Here's how the part is built. I have some questions about the finished solid (model axes, mm). Give positions to 0.01 mm unless a question says otherwise; leave off trailing zeros. Order: outer loops, then holes, each group sorted by start corner. A loop starts at its lowest first (then second) coordinate and runs counter-clockwise, first axis right, second up. Notation, with made-up numbers: (12, 68.5) - (52, 68.5) arc R18 ccw to (52, 72.5) - close; hole circle Ø7 at (80.25, -22). An arc over 180 degrees is marked (long way). One line per question, with ' | ' between items.
from build123d import *

# Parameters (mm, degrees)
F0_W     = 111.695483
F0_H     = 93.271062
F1_DEPTH = 38.75114
F2_SIZE  = 12.7
F3_W     = 73.332176
F3_H     = 55.99878
F4_DEPTH = 6.398048


with BuildPart() as f1:
    # F0 (on Top) → F1 (new body)
    with BuildSketch(Plane.XY):
        with Locations((12.841567, 46.635531)):
            Rectangle(F0_W, F0_H)
    extrude(amount=-F1_DEPTH)

    # F2
    f2_edges = [f1.edges().sort_by_distance(p)[0] for p in [
        (68.689309, 46.635531, -38.75114),
    ]]
    chamfer(f2_edges, length=F2_SIZE)

    # F3 (on face) → F4 (join)
    with BuildSketch(Plane(origin=(0, 0, -38.75114), x_dir=(1, 0, 0), z_dir=(0, 0, -1))):
        with Locations((-1.400314, -35.273772)):
            Rectangle(F3_W, F3_H)
    extrude(amount=F4_DEPTH)


solid = f1.part
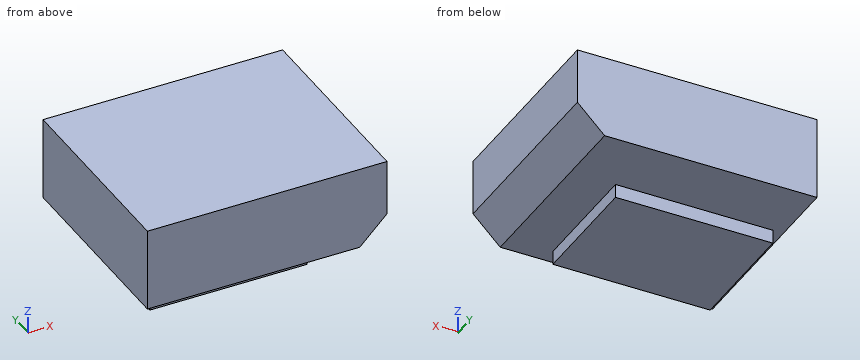
1) I'm going to push flat-ended pins straight in: P1, Ø12, axis at y = 43, z = -39.5, coming from the +X side; P2, Ø5, axis at x = -17, z = -43.5, coming from the +Y side; P3, Ø3, axis at y = 27, z = -41.5, coming from the +X side. Where does each tip first touch, or does it pass through?
Model answer:
P1: stops at x = 61.24 | P2: stops at y = 63.27 | P3: stops at x = 35.27
2) Please list where these lines run through material, in increasing order: L1, parallel to Y at x = 34, z = -41; L2, parallel to Z at x = 42.5, y = 40; L3, parallel to X at y = 47, z = -41.
Model answer:
L1: y = 7.27 to 63.27 | L2: z = -38.75 to 0 | L3: x = -38.07 to 35.27
3) I want a section at A-A (y = 10). List the corners of the cut face in (x, z) for me.
Model answer:
outline: (-43.01, -38.75) - (-38.07, -38.75) - (-38.07, -45.15) - (35.27, -45.15) - (35.27, -38.75) - (55.99, -38.75) - (68.69, -26.05) - (68.69, 0) - (-43.01, 0) - close
4) I want a section at D-D (y = 84). List the corners of the cut face in (x, z) for me, plus the area to 3 significant figures.
Model answer:
outline: (-43.01, -38.75) - (55.99, -38.75) - (68.69, -26.05) - (68.69, 0) - (-43.01, 0) - close | area: 4,250 mm2
5) I want a section at B-B (x = 12.5). List the corners of the cut face in (y, z) for me, plus the area to 3 significant figures.
Model answer:
outline: (0, -38.75) - (7.27, -38.75) - (7.27, -45.15) - (63.27, -45.15) - (63.27, -38.75) - (93.27, -38.75) - (93.27, 0) - (0, 0) - close | area: 3,970 mm2
6) I want a section at C-C (z = -31). List the corners of the cut face in (x, y) for me.
Model answer:
outline: (-43.01, 0) - (63.74, 0) - (63.74, 93.27) - (-43.01, 93.27) - close
